Geometry check sheet. Reference: the model listing, model coordinates, mm. Face numbers are marked on the shaded views. Give positions to 0.01 mm unless a question says otherwise; leave off trailing zeros. Write each loop counter-clockwise with the first axis right and the second up, starting at its lowest first coordinate (ties: lowest second). Pieces come first, ordered by that corner, then holes. Notation, with made-up numbers: (-19, 85.5) -> (-7, 85.5) arc R26 ccw to (-7, 110.5) -> close; hole circle Ø3 at (28.5, 63). An arc over 180 degrees is marked (long way). One line per item, written item: value.
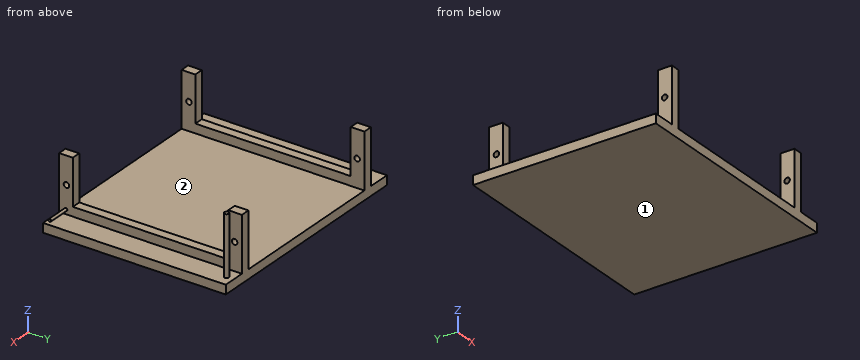
from build123d import *

# Parameters (mm, degrees)
ESQUISSE1_W             = 250
ESQUISSE1_H             = 200
BOSS_EXTRU_1_DEPTH      = 10
ESQUISSE2_W             = 10
ESQUISSE2_H             = 200
BOSS_EXTRU_2_DEPTH      = 60
ESQUISSE3_R             = 3
ESQUISSE3_W             = 50
ESQUISSE3_H             = 170
ENL_V_MAT_EXTRU_1_DEPTH = 226
ESQUISSE4_R             = 2.5
BOSS_EXTRU_5_DEPTH      = 65
ESQUISSE8_R             = 1.5
BOSS_EXTRU_8_DEPTH      = 25


with BuildPart() as part:
    # Esquisse1 → Boss.-Extru.1 (new body)
    with BuildSketch(Plane.XY):
        with Locations((125, -100)):
            Rectangle(ESQUISSE1_W, ESQUISSE1_H)
    extrude(amount=BOSS_EXTRU_1_DEPTH)

    # Esquisse2 → Boss.-Extru.2 (add)
    with BuildSketch(Plane.XY.offset(10)):
        with Locations((30, -100)):
            Rectangle(ESQUISSE2_W, ESQUISSE2_H)
        with Locations((220, -100)):
            Rectangle(ESQUISSE2_W, ESQUISSE2_H)
    extrude(amount=BOSS_EXTRU_2_DEPTH)

    # Esquisse3 → Enlèv. mat.-Extru.1 (cut, through all)
    with BuildSketch(Plane(origin=(225, 0, 0), x_dir=(0, 0, -1), z_dir=(1, 0, 0))):
        with Locations((-40, -192)):
            Circle(ESQUISSE3_R)
        with Locations((-40, -8)):
            Circle(ESQUISSE3_R)
        with Locations((-45, -100)):
            Rectangle(ESQUISSE3_W, ESQUISSE3_H)
    extrude(amount=-ENL_V_MAT_EXTRU_1_DEPTH, mode=Mode.SUBTRACT)

    # Esquisse4 → Boss.-Extru.5 (add)
    with BuildSketch(Plane.XY.offset(10)):
        with Locations((237.5, -8)):
            Circle(ESQUISSE4_R)
    extrude(amount=BOSS_EXTRU_5_DEPTH)

    # Esquisse8 → Boss.-Extru.8 (add)
    with BuildSketch(Plane(origin=(225, 0, 0), x_dir=(0, 0, -1), z_dir=(1, 0, 0))):
        with Locations((-15, -192.5)):
            Circle(ESQUISSE8_R)
    extrude(amount=BOSS_EXTRU_8_DEPTH)


solid = part.part
1) Sectioned sample at A-A on z = 53. Record the cut outline in (x, y), plus the area to 3 significant figures.
Verdict:
outline: (25, -200) -> (35, -200) -> (35, -185) -> (25, -185) -> close; (25, -15) -> (35, -15) -> (35, 0) -> (25, 0) -> close; (215, -200) -> (225, -200) -> (225, -185) -> (215, -185) -> close; (215, -15) -> (225, -15) -> (225, 0) -> (215, 0) -> close; circle Ø5 at (237.5, -8)
area: 620 mm^2
2) Depth check by flat-ended pin: pin 1 Ø11 at (x, y) = (31.5, -190.5) entering from +Z; pin 2 Ø5 at (x, y) = (175.5, -160.5) entering from +Z; pin 3 Ø7 at (y, z) = (-8, 40) entering from -X. Enter the tip coordinate at first touch or a pass-through.
Verdict:
pin 1: z = 70
pin 2: z = 10
pin 3: x = 25
3) Sectioned sample at B-B on y = -116.5. Record the cut outline in (x, z), plus the area to 3 significant figures.
Verdict:
outline: (0, 0) -> (250, 0) -> (250, 10) -> (225, 10) -> (225, 20) -> (215, 20) -> (215, 10) -> (35, 10) -> (35, 20) -> (25, 20) -> (25, 10) -> (0, 10) -> close
area: 2,700 mm^2
4) Sectioned sample at C-C on x = 41. Record the cut outline in (y, z), plus the area to 3 significant figures.
Verdict:
outline: (-200, 0) -> (0, 0) -> (0, 10) -> (-200, 10) -> close
area: 2,000 mm^2
5) Mould release check, pull along X, two halves, no side actions. Record for the marked faces 1 and 2: released by +X, released by -X, zero draft, split by the parting line, or undercut.
Verdict:
face 1: zero draft
face 2: undercut
6) Scan lines: probe 1 along Y at (x, z) = (30.75, 40); probe 2 along X at (y, z) = (-131, 18.5); probe 3 along Z at (x, y) = (28, -192). Record each from-to range of solid material in increasing order.
Verdict:
probe 1: -200 to -195, -189 to -185, -15 to -11, -5 to 0
probe 2: 25 to 35, 215 to 225
probe 3: 0 to 37, 43 to 70
